Verification items for the finished model (mm, model axes). Round coordinates to 2 decimals unless told otherwise and drop trailing zeros. Write each loop counter-clockwise with the first axis right and the second up, starting at its lowest first coordinate (ties: lowest second). Pieces come first, ordered by that corner, then holes. Notation, with made-up numbers: (41.25, -17.5) -> (80.25, -17.5) arc R11 ccw to (80.25, -11.5) -> close; hole circle Ø6 at (36.5, 19). An arc over 180 degrees is marked (long way). Answer as a JSON object with one key per item and string values. Group by question number.
(1) Draft check along Y on faces 1 (the face through (-12, 0, -7)), 2 (the face through (-13, 3, 0)), 3 (the face through (-12.522, 13.333, -7.139)), 4 (the face through (-12.59, 10.98, -6.69)). Enter one of: released by +Y, released by -Y, zero draft, split by the parting line, or undercut.
(2) Sectioned sample at B-B on y = 1. Record the cut outline in (x, z) (3 decimals), and give its area (3 significant figures).
(3) Sectioned sample at C-C on x = -9.5. Count the separate pieces of the cut face and the enclosed holes in it, and give its area (3 significant figures).
(4) Sectioned sample at D-D on z = -5. Record the cut outline in (x, y).
(5) Gauge pin test, flat ends, axial feed: pin 1 Ø2 at (y, z) = (11.684, -6.985) entering from -X; pin 2 Ø6 at (y, z) = (3.18, -10.48) entering from -X; pin 3 Ø3 at (x, z) = (-9.5, -9) entering from +Y. Record the tip position at first contact, or that the pin passes through.
(6) Sectioned sample at A-A on z = -2.5. Record the cut outline in (x, y), and give its area (3 significant figures).
(7) Scan lines: L1, parallel to Z at x = -15, y = 4.5; L2, parallel to Z at x = -16.75, y = 1.25; L3, parallel to Y at x = 0.75, z = -5.5. Record each from-to range of solid material in increasing order. Write a range as from..to.
```python
from build123d import *
from build123d.topology import SkipClean

# Parameters (mm, degrees)
SKETCH1_W                             = 25.4
SKETCH1_H                             = 13.97
DEPTH_A_DEPTH                         = 6.35
ROUND_EXTRUDE_DEPTH                   = 25.4
ANGLE_CUT_DEPTH                       = 32.908355097
STRING_HOLE_R                         = 0.762
STRING_HOLE_CUT_DEPTH                 = 32.908355097
ELASTIC_HOLE_CUT_DEPTH                = 32.908355097
ELASTIC_HOLE_CUT_DEPTH_BACK           = 32.908355097
ELASTIC_HOLES_R                       = 2.54
GUIDE_OUTIE_EXTRUDE_REACH             = 33.908
SKETCH7_R                             = 2.54
ELASTIC_HOLE_CUT_ON_GUIDE_OUTIE_DEPTH = 32.908355097
GUIDE_INNIE_CUT_DEPTH                 = 32.908355141


with BuildPart() as part:
    # Sketch1 → depth a (new body)
    with BuildSketch(Plane(origin=(0, 0, 0), x_dir=(1, 0, 0), z_dir=(0, 1, 0))):
        with Locations((-12.7, 6.985)):
            Rectangle(SKETCH1_W, SKETCH1_H)
    extrude(amount=DEPTH_A_DEPTH)

    # Sketch4 → round extrude (add)
    with BuildSketch(Plane(origin=(0, 0, 0), x_dir=(0, 0, -1), z_dir=(1, 0, 0))):
        with BuildLine():
            Line((0, 6.35), (13.97, 6.35))
            ThreePointArc((13.97, 6.35), (6.985, 13.335), (0, 6.35))
        make_face()
    extrude(amount=-ROUND_EXTRUDE_DEPTH)

    # Sketch5 → angle cut (cut, through all)
    with BuildSketch(Plane.XY):
        Polygon((0, 6.35), (0, 13.335), (-6.985, 13.335), align=None)
        Polygon((-25.4, 6.35), (-25.4, 13.335), (-18.415, 13.335), align=None)
    extrude(amount=-ANGLE_CUT_DEPTH, mode=Mode.SUBTRACT)

    # string hole → string hole cut (cut, through all)
    with BuildSketch(Plane(origin=(0, 0, 0), x_dir=(0, 0, -1), z_dir=(1, 0, 0))):
        with Locations(Location((6.985, 11.684, 0), (0, 0, 270))):
            Circle(STRING_HOLE_R)
    extrude(amount=-STRING_HOLE_CUT_DEPTH, mode=Mode.SUBTRACT)

    # elastic holes → elastic hole cut (cut, two sides: drawn at the far end of the back side and taken through both)
    with BuildSketch(Plane(origin=(0, 0, 0), x_dir=(0, 0, -1), z_dir=(1, 0, 0)).offset(-ELASTIC_HOLE_CUT_DEPTH_BACK)):
        with Locations((3.4925, 3.175)):
            Circle(ELASTIC_HOLES_R)
        with Locations(Location((10.4775, 3.175, 0), (0, 0, 180))):
            Circle(ELASTIC_HOLES_R)
    extrude(amount=ELASTIC_HOLE_CUT_DEPTH + ELASTIC_HOLE_CUT_DEPTH_BACK, mode=Mode.SUBTRACT)

    # guide outie extrude: up to this plane
    guide_outie_extrude_end = Plane(origin=(-6.985, 13.335, -13.97), z_dir=(-0.7071067811865512, -0.7071067811865439, 0))
    # guide outie → guide outie extrude (add, up to the surface)
    with BuildSketch(Plane(origin=(0, 0, 0), x_dir=(1, 0, 0), z_dir=(0, 1, 0)), mode=Mode.PRIVATE) as guide_outie_extrude_sk1:
        with BuildLine():
            Line((0, 13.97), (0, 0))
            ThreePointArc((0, 0), (2.781966725, 6.985), (0, 13.97))
        make_face()
    guide_outie_extrude_tool1 = split(extrude(guide_outie_extrude_sk1.sketch, amount=GUIDE_OUTIE_EXTRUDE_REACH, mode=Mode.PRIVATE), bisect_by=guide_outie_extrude_end, keep=Keep.BOTH, mode=Mode.PRIVATE)
    add(guide_outie_extrude_tool1.solids().sort_by_distance((1.126975, 0, -6.985))[0])

    # Sketch7 → elastic hole cut on guide outie (cut, through all)
    with SkipClean():  # the faces are left unmerged after this step: merging them gives an invalid solid
        with BuildSketch(Plane.ZY):
            with Locations(Location((-3.4925, 3.175, 0), (0, 0, 180))):
                Circle(SKETCH7_R)
            with Locations(Location((-10.4775, 3.175, 0), (0, 0, 133.366502627))):
                Circle(SKETCH7_R)
        extrude(amount=-ELASTIC_HOLE_CUT_ON_GUIDE_OUTIE_DEPTH, mode=Mode.SUBTRACT)

    # guide innie → guide innie cut (cut, through all)
    with SkipClean():  # the faces are left unmerged after this step: merging them gives an invalid solid
        with BuildSketch(Plane(origin=(0, 0, 0), x_dir=(1, 0, 0), z_dir=(0, 1, 0))):
            with BuildLine():
                Line((-25.4, 13.97), (-25.4, 0))
                ThreePointArc((-25.4, 0), (-22.618033275, 6.985), (-25.4, 13.97))
            make_face()
        extrude(amount=GUIDE_INNIE_CUT_DEPTH, mode=Mode.SUBTRACT)


solid = part.part
```
Computed values:
{
 "1": {"face 1": "released by -Y", "face 2": "zero draft", "face 3": "released by +Y", "face 4": "undercut"},
 "2": {"outline": "(-25.4, -13.97) -> (0, -13.97) arc R10.16 ccw to (1.574, -11.789) -> (-23.826, -11.789) arc R10.16 cw to start; (-25.4, 0) arc R10.16 cw to (-23.826, -2.181) -> (1.574, -2.181) arc R10.16 ccw to (0, 0) -> close; (-22.855, -9.166) -> (2.545, -9.166) arc R10.16 ccw to (2.545, -4.804) -> (-22.855, -4.804) arc R10.16 cw to start", "area": "222 mm2"},
 "3": {"separate pieces": "1", "enclosed holes": "3", "area": "123 mm2"},
 "4": {"outline": "(-22.81, 0) -> (2.59, 0) -> (2.59, 1.13) -> (-22.81, 1.13) -> close; (-22.81, 5.22) -> (1.13, 5.22) -> (-6.7, 13.05) -> (-18.7, 13.05) -> (-22.81, 8.94) -> close"},
 "5": {"pin 1": "x = -21.07", "pin 2": "x = -24.97", "pin 3": "y = 13.32"},
 "6": {"outline": "(-23.66, 0) -> (1.74, 0) -> (1.74, 0.84) -> (-23.66, 0.84) -> close; (-23.66, 5.51) -> (0.84, 5.51) -> (-5.35, 11.7) -> (-20.05, 11.7) -> (-23.66, 8.09) -> close", "area": "147 mm2"},
 "7": {"L1": "-13.97..-12.64, -8.31..-5.66, -1.33..0", "L2": "-13.97..-12.13, -8.82..-5.15, -1.84..0", "L3": "0..1.62, 4.73..5.6"}
}
